Verification items for the finished model (mm, model axes). Face numbers are marked on the shaded views. A direction names the side the tool comes from. Round coordinates to 2 decimals unless told otherwise and drop trailing zeros. Order: outer loops, then holes, each group sorted by start corner. A loop starts at its lowest first (then second) coordinate and runs counter-clockwise, first axis right, second up. Notation, with made-up numbers: M 61,-9 L 69,-9 A37 cw 69,30 Z; hole C 59.25,18.5 d6. An arc over 180 degrees is marked long. Use one line per item in the form item = value. Start each with the question number.
Item 1: Thickness scan on probe 1 along X at (y, z) = (1.95, 1.1); probe 2 along Y at (x, z) = (7.5, -0.1); probe 3 along Z at (x, y) = (-2.5, 0.5). Record the ranges inside material, lowest first. Write a range as [from, to].
Item 2: Cross-section at B-B on x = -1.5. Enter the section's corners in (y, z), then the cut area to 3 significant figures.
Item 3: Cross-section at A-A on x = 8.5. Enter the section's corners in (y, z), then the cut area to 3 significant figures.
Item 4: Go/stop test with flat-tipped pins: pin 1 Ø1.5 at (x, z) = (6, 0) entering from +Y; pin 2 Ø3 at (x, y) = (6.5, -2) entering from +Z. Record where each tip stops, or that it passes through.
Item 5: Tool access check on the marked faces 1, 2 and 3. Record the directions out of +Z, -Z, +X, -X, +Y, -Y that give a thin tool (end or side, any length) a straight path to the whole face; none if there is none.
Autodesk Inventor part; units mm, degrees
ref_plane "Work Plane1" through (29, 0, 0) normal (0, -1, 0) x (1, 0, 0)
ref_plane "YZ Plane" through (0, 0, 0) normal (1, 0, 0) x (0, 1, 0)
ref_plane "XZ Plane" through (0, 0, 0) normal (0, 1, 0) x (-1, 0, 0)
sketch "Sketch1" plane through (0, 0, 0) normal (0, 0, 1) x (1, 0, 0)
  line L0 (-0.9567, 0) -> (9.525, 0)
  line L1 (9.525, 0) -> (9.525, 1.7526)
  line L2 (9.525, 1.7526) -> (1.9844, 1.7526)
  line L3 (1.9844, 1.7526) -> (0.0001, 1.7526)
  line L4 (0.0001, 1.7526) -> (0, 1.7526)
  line L5 (0, 1.7526) -> (0, 2.8702)
  line L6 (0, 2.8702) -> (-3.5052, 2.8702)
  line L7 (-3.5052, 2.8702) -> (-3.5052, 1.5985)
  line L8 (-3.5052, 1.5985) -> (-1.8796, 1.5985)
  line L9 (-1.8796, 1.5985) -> (-0.9567, 0)
  line L10 (-6.1112, 0) -> (12.131, 0)
  line L11 (0, -0.574) -> (0, 3.4442)
  line L12 (1.9844, 1.7526) -> (0, 1.7526) construction
  dimension "d1" = 7.5405
  dimension "d2" = 1.9844
  dimension "d3" = 3.5052
  dimension "d4" = 1.6256
  dimension "d5" = 60
  dimension "d6" = 3.5052
  dimension "d7" = 3.5052
  dimension "d8" = 3.1969
  dimension "d9" = 5.7404
  dimension "d26" = 9.525
revolve "Body" add sketch "Sketch1" angle 360 about axis through (-0.9567, 0, 0) along (1, 0, 0)
sketch "Sketch2" plane through (-3.5052, 0, 0) normal (-1, 0, 0) x (0, 0, 1)
  circle A0 centre (0, 0) radius 1.5985
  line L0 (0, -4.0183) -> (0, 4.0183)
  line L1 (-4.0183, 0) -> (4.0183, 0)
  line L2 (1.5985, 0) -> (0.7992, -1.3843)
  line L3 (0.7992, -1.3843) -> (-0.7992, -1.3843)
  line L4 (-0.7992, -1.3843) -> (-1.5985, 0)
  line L5 (-1.5985, 0) -> (-0.7992, 1.3843)
  line L6 (-0.7992, 1.3843) -> (0.7992, 1.3843)
  line L7 (0.7992, 1.3843) -> (1.5985, 0)
extrude "Slot" add sketch "Sketch2" against normal up to next contours L7 A0 | A0 L2 | L6 L0 A0 | A0 L0 L3 | L0 L6 A0 | A0 L3 L0 | L4 A0 | A0 L5
fillet "Fillet1" radius 0.3302 1 edges at (-3.5052, -2.8702, 0)
thread "Thread"
chamfer "Chamfer1" distance 0.4724 distance2 0.4724 1 edges at (9.525, -1.7526, 0) measured on face at (9.525, 0.5173, 0.2715)
ref_plane "Work Plane1" through (29, 0, 0) normal (0, -1, 0) x (1, 0, 0)
fillet "Fillet2" radius 0.127 1 edges at (0.0001, -1.7526, 0)
equation "\"d1\" = GEL"
equation "\"d3\" = KOH"
equation "\"d4\" = INTI"
equation "\"d6\" = GD"
equation "\"d7\" = BDM"
equation "\"d8\" = 1.1547 * SW"
equation "\"d9\" = KOD"
equation "\"d26\" = NLG"
equation "\"d30\" = R"
equation "\"d17\" = RR"
equation "\"d13\" = GEL"
equation "\"d15\" = -0.5 * SPD + 0.5 * GD"
equation "\"d16\" = GUL"
equation "\"GD\" = 3.5052"
equation "\"NLG\" = 9.525"
equation "\"GEL\" = 7.54055"
equation "\"KOD\" = 5.7404"
equation "\"KOH\" = 3.5052"
equation "\"INTI\" = 1.6256"
equation "\"GAL\" = 1.98425"
equation "\"GUL\" = 0.47244"
equation "\"BDM\" = 3.5052"
equation "\"SW\" = 2.7686"
equation "\"RR\" = 0.3302"
equation "\"SPD\" = 2.56032"
equation "\"R\" = 0.127"
equation "\"PHH\" = 0.127"
equation "\"GD1\" = SPD"
equation "\"THREADDIA\" = 3.5052"
equation "\"FAWI\" = 45deg"
equation "\"KOH1\" = 3.1496"
equation "\"NND\" = 3.5052"
equation "\"TOA\" = 30deg"
equation "\"E0\" = 1.155 * SW"
properties part number "ANSI B18.3 - No. 6 - 32 UNC - 3/8 HS HCS" material "Steel, Alloy"
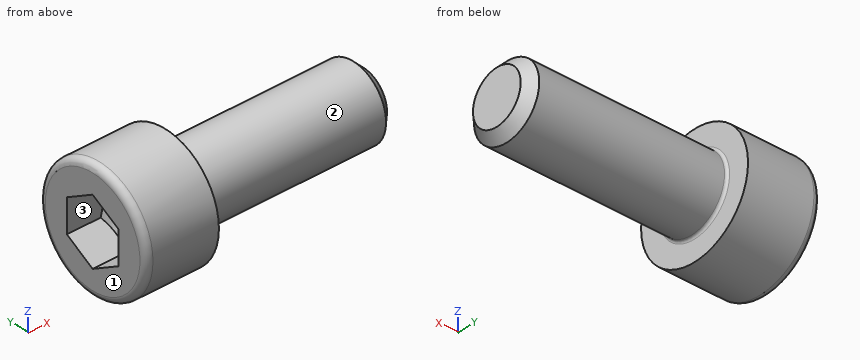
Output values:
q1.probe_1 = [-3.51, 0]
q1.probe_2 = [-1.75, 1.75]
q1.probe_3 = [-2.83, -1.31], [1.31, 2.83]
q2.outline = C 0,0 d5.74; hole C 0,0 d1.88
q2.area = 23.1 mm2
q3.outline = C 0,0 d3.51
q3.area = 9.65 mm2
q4.pin_1 = 1.75
q4.pin_2 = 1.68
q5.face_1 = +Z, -Z, -X, +Y, -Y
q5.face_2 = +X
q5.face_3 = -X
